```python
from build123d import *

# Parameters (mm, degrees)
SKETCH2_R               = 91.355
SKETCH2_R_2             = 86.355
BOSS_EXTRUDE1_DEPTH     = 15
SKETCH5_W               = 90
SKETCH5_H               = 30
CUT_EXTRUDE1_DEPTH      = 131.063338609
CUT_EXTRUDE2_DEPTH      = 131.063338609
CUT_EXTRUDE2_DEPTH_BACK = 131.063338609
SKETCH6_W               = 138.372037672
SKETCH6_H               = 21.288005796


with BuildPart() as part:
    # Sketch2 → Boss-Extrude1 (new, symmetric)
    with BuildSketch(Plane(origin=(0, 0, 0), x_dir=(1, 0, 0), z_dir=(0, 1, 0))):
        with Locations(Location((0, 0, 0), (0, 0, 270))):
            Circle(SKETCH2_R)
        with Locations(Location((0, 0, 0), (0, 0, 270))):
            Circle(SKETCH2_R_2, mode=Mode.SUBTRACT)
    extrude(amount=BOSS_EXTRUDE1_DEPTH, both=True)

    # Sketch5 → Cut-Extrude1 (cut, through all)
    with BuildSketch(Plane.XY):
        Rectangle(SKETCH5_W, SKETCH5_H)
    extrude(amount=-CUT_EXTRUDE1_DEPTH, mode=Mode.SUBTRACT)

    # Sketch6 → Cut-Extrude2 (cut, two sides: drawn at the far end of the back side and taken through both)
    with BuildSketch(Plane(origin=(0, 0, 0), x_dir=(0, 0, -1), z_dir=(1, 0, 0)).offset(-CUT_EXTRUDE2_DEPTH_BACK)):
        Rectangle(SKETCH6_W, SKETCH6_H)
    extrude(amount=CUT_EXTRUDE2_DEPTH + CUT_EXTRUDE2_DEPTH_BACK, mode=Mode.SUBTRACT)


solid = part.part
```
CAD build for the part. Positions are in the model's coordinates, mm. A direction names the side the tool comes from. Round coordinates to 2 decimals unless told otherwise and drop trailing zeros. Order: outer loops, then holes, each group sorted by start corner. A loop starts at its lowest first (then second) coordinate and runs counter-clockwise, first axis right, second up. Notation, with made-up numbers: (70, 48.5) - (114, 48.5) arc R25 ccw to (114, 72.5) - close; hole circle Ø1 at (23, 65). An arc over 180 degrees is marked (long way). Answer in a Markdown table with one row per item. Add a question column.
(1) 3-axis set-ups, long thin cutter, end or side, ignore diameter. For faces 1 (the face through (-45, 0, -77)), 2 (the face through (0, 15, 88)), 3 (the face through (56, 0, 69.186)): which of +Z, -Z, +X, -X, +Y, -Y reach the whole face in a straight line?
(2) Probe L1, parallel to Z at x = -2, y = 6.75; L2, parallel to X at y = 12.25, z = 65; L3, parallel to Z at x = 0, y = 3 (3 decimals). List the from-to ranges inside material, lowest first. Write a range as [from, to].
(3) Band-saw the part on B-B on z = 0. List the corners of the cut face in (x, y) (3 decimals).
(4) Drop flat-ended pins along their axis: pin 1 Ø6.5 at (y, z) = (6, -76) entering from +X; pin 2 Ø6.5 at (x, y) = (-56.5, 1.5) entering from -Z; pin 3 Ø1.5 at (x, y) = (63.5, 9.5) entering from +Z; pin 4 Ø2.5 at (x, y) = (57, -4) entering from +Z. Give the stop position or say it passes through.
(5) Mould opens along Z. For faces 4 (the face through (45, 0, -77)), 5 (the face through (-56, 0, 69.186)), 6 (the face through (-3.359, 0.21, 91.293)) say: +Z half, -Z half, draft (parallel to the pull), parting line (faces both ways), or undercut.
(6) Band-saw the part on A-A on y = -8.5. List the corners of the cut face in (x, z) (3 decimals).
(7) Band-saw the part on C-C on x = -64.5. List the corners of the cut face in (y, z).
(8) Band-saw the part on D-D on x = 49. List the corners of the cut face in (y, z).
Data:
| question | item | result |
|---|---|---|
| 1 | face 1 | -Z, +Y, -Y |
| 1 | face 2 | +Z, -Z, +X, -X, +Y |
| 1 | face 3 | +X, -X |
| 2 | L1 | z = [86.33, 91.33] |
| 2 | L2 | x = [-64.19, -56.85], [56.85, 64.19] |
| 2 | L3 | z = [86.355, 91.355] |
| 3 | outline | (-91.355, -15) - (-86.355, -15) - (-86.355, -10.644) - (-91.355, -10.644) - close; (-91.355, 10.644) - (-86.355, 10.644) - (-86.355, 15) - (-91.355, 15) - close; (86.355, -15) - (91.355, -15) - (91.355, -10.644) - (86.355, -10.644) - close; (86.355, 10.644) - (91.355, 10.644) - (91.355, 15) - (86.355, 15) - close |
| 4 | pin 1 | stops at x = 55.26 |
| 4 | pin 2 | stops at z = -74.23 |
| 4 | pin 3 | passes through |
| 4 | pin 4 | stops at z = 72.37 |
| 5 | face 4 | draft |
| 5 | face 5 | undercut |
| 5 | face 6 | parting line |
| 6 | outline | (-59.658, -69.186) arc R91.355 ccw to (-45, -79.503) - (-45, -73.703) arc R86.355 cw to (-51.677, -69.186) - close; (-59.658, 69.186) - (-51.677, 69.186) arc R86.355 cw to (51.677, 69.186) - (59.658, 69.186) arc R91.355 ccw to start; (45, -79.503) arc R91.355 ccw to (59.658, -69.186) - (51.677, -69.186) arc R86.355 cw to (45, -73.703) - close |
| 7 | outline | (-15, -64.7) - (-10.64, -64.7) - (-10.64, -57.42) - (-15, -57.42) - close; (-15, 57.42) - (-10.64, 57.42) - (-10.64, 64.7) - (-15, 64.7) - close; (10.64, -64.7) - (15, -64.7) - (15, -57.42) - (10.64, -57.42) - close; (10.64, 57.42) - (15, 57.42) - (15, 64.7) - (10.64, 64.7) - close |
| 8 | outline | (-15, -77.1) - (15, -77.1) - (15, -71.11) - (-15, -71.11) - close; (-15, 71.11) - (15, 71.11) - (15, 77.1) - (-15, 77.1) - close |
